CAD build for the part. Positions are in the model's coordinates, mm. Face numbers are marked on the shaded views. A direction names the side the tool comes from. Give positions to 0.01 mm unless a question says otherwise; leave off trailing zeros. Loops run counter-clockwise (first coordinate to the right, second up) from the corner with the lowest first, then second, coordinate; pieces in that order, holes last. Notation, with made-up numbers: (3, 20.5) - (22, 20.5) arc R19 cw to (22, 26.5) - close; hole circle Ø7 at (80, 20.25). An arc over 180 degrees is marked (long way). Return JSON: item names as keys, results as strings.
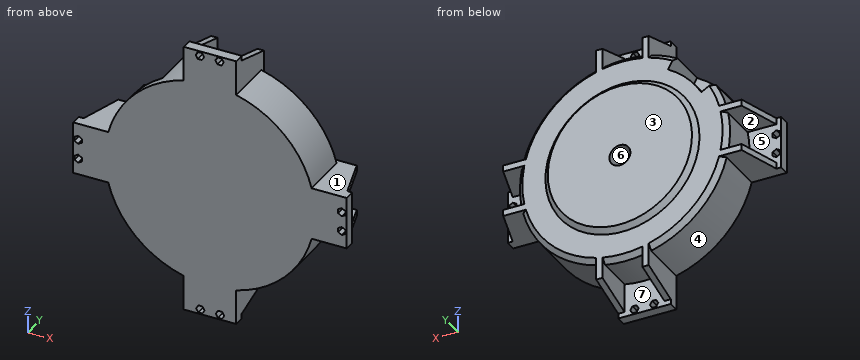
from build123d import *

# Parameters (mm, degrees)
BOSS_EXTRUDE1_DEPTH                      = 37.5
SKETCH4_W                                = 3.5
SKETCH4_H                                = 30
CUT_EXTRUDE1_DEPTH                       = 37.5
SKETCH7_W                                = 3.5
SKETCH7_H                                = 30
CUT_EXTRUDE3_DEPTH                       = 157.454118834
CUT_EXTRUDE4_START                       = -30
CUT_EXTRUDE4_DEPTH                       = 30
CHAMFER1_SIZE                            = 3.5
CUT_EXTRUDE5_DEPTH                       = 157.454118834
MIRROR4_AT_THE_SECOND_PLANE_COPY_1_DEPTH = 157.454118834
CUT_EXTRUDE6_DEPTH                       = 157.454118834
CUT_EXTRUDE7_DEPTH                       = 144.057956088
CUT_EXTRUDE7_DEPTH_BACK                  = 30
SKETCH14_R                               = 55
BOSS_EXTRUDE3_DEPTH                      = 3.5
CHAMFER2_SIZE                            = 3.5
SKETCH15_R                               = 7.5
CUT_EXTRUDE8_DEPTH                       = 25


with BuildPart() as part:
    # Sketch2 → Boss-Extrude1 (new body)
    with BuildSketch(Plane(origin=(0, 0, 0), x_dir=(1, 0, 0), z_dir=(0, 1, 0))):
        with BuildLine():
            Line((97.62, 0), (97.62, 18.75))
            Line((97.62, 18.75), (72.618437741, 18.75))
            ThreePointArc((72.618437741, 18.75), (53.033008589, 53.033008589), (18.75, 72.618437741))
            Line((18.75, 72.618437741), (18.75, 97.62))
            Line((18.75, 97.62), (0, 97.62))
            Line((0, 97.62), (-18.75, 97.62))
            Line((-18.75, 97.62), (-18.75, 72.618437741))
            ThreePointArc((-18.75, 72.618437741), (-53.033008589, 53.033008589), (-72.618437741, 18.75))
            Line((-72.618437741, 18.75), (-97.62, 18.75))
            Line((-97.62, 18.75), (-97.62, 0))
            Line((-97.62, 0), (-97.62, -18.75))
            Line((-97.62, -18.75), (-72.618437741, -18.75))
            ThreePointArc((-72.618437741, -18.75), (-53.033008589, -53.033008589), (-18.75, -72.618437741))
            Line((-18.75, -72.618437741), (-18.75, -97.62))
            Line((-18.75, -97.62), (0, -97.62))
            Line((0, -97.62), (18.75, -97.62))
            Line((18.75, -97.62), (18.75, -72.618437741))
            ThreePointArc((18.75, -72.618437741), (53.033008589, -53.033008589), (72.618437741, -18.75))
            Line((72.618437741, -18.75), (97.62, -18.75))
            Line((97.62, -18.75), (97.62, 0))
        make_face()
        Polygon((8.323894459, -96.71614814), (5.323896931, -96.72), (3.820562359, -94.12385186), (5.317225314, -91.52385186), (8.317222841, -91.52), (9.820557413, -94.11614814), align=None, mode=Mode.SUBTRACT)
        Polygon((-5.682777159, -96.72), (-4.179442587, -94.12385186), (-5.676105541, -91.52385186), (-8.676103069, -91.52), (-10.179437641, -94.11614814), (-8.682774686, -96.71614814), align=None, mode=Mode.SUBTRACT)
        Polygon((-96.71614814, -8.323894459), (-96.72, -5.323896931), (-94.12385186, -3.820562359), (-91.52385186, -5.317225314), (-91.52, -8.317222841), (-94.11614814, -9.820557413), align=None, mode=Mode.SUBTRACT)
        Polygon((96.72, -5.682777159), (94.12385186, -4.179442587), (91.52385186, -5.676105541), (91.52, -8.676103069), (94.11614814, -10.179437641), (96.71614814, -8.682774686), align=None, mode=Mode.SUBTRACT)
        Polygon((96.71614814, 8.323894459), (96.72, 5.323896931), (94.12385186, 3.820562359), (91.52385186, 5.317225314), (91.52, 8.317222841), (94.11614814, 9.820557413), align=None, mode=Mode.SUBTRACT)
        Polygon((-96.72, 5.682777159), (-94.12385186, 4.179442587), (-91.52385186, 5.676105541), (-91.52, 8.676103069), (-94.11614814, 10.179437641), (-96.71614814, 8.682774686), align=None, mode=Mode.SUBTRACT)
        Polygon((-8.323894459, 96.71614814), (-5.323896931, 96.72), (-3.820562359, 94.12385186), (-5.317225314, 91.52385186), (-8.317222841, 91.52), (-9.820557413, 94.11614814), align=None, mode=Mode.SUBTRACT)
        Polygon((5.682777159, 96.72), (4.179442587, 94.12385186), (5.676105541, 91.52385186), (8.676103069, 91.52), (10.179437641, 94.11614814), (8.682774686, 96.71614814), align=None, mode=Mode.SUBTRACT)
    extrude(amount=BOSS_EXTRUDE1_DEPTH)

    # Sketch4 → Cut-Extrude1 (cut)
    with BuildSketch(Plane.XY.offset(18.75)):
        with Locations((-95.87, 22.5)):
            Rectangle(SKETCH4_W, SKETCH4_H)
    cut_extrude1 = extrude(amount=-CUT_EXTRUDE1_DEPTH, mode=Mode.SUBTRACT)

    # Sketch7 → Cut-Extrude3 (cut, through all)
    with BuildSketch(Plane(origin=(18.75, 0, 0), x_dir=(0, 0, -1), z_dir=(1, 0, 0))):
        with Locations((-95.87, 22.5)):
            Rectangle(SKETCH7_W, SKETCH7_H)
    cut_extrude3 = extrude(amount=-CUT_EXTRUDE3_DEPTH, mode=Mode.SUBTRACT)

    # Mirror1: Cut-Extrude3 across plane
    add(cut_extrude3.mirror(Plane.XY), mode=Mode.SUBTRACT)

    # Mirror2: Cut-Extrude1 across plane
    add(cut_extrude1.mirror(Plane.ZY), mode=Mode.SUBTRACT)

    # Sketch8 → Cut-Extrude4 (cut)
    with BuildSketch(Plane(origin=(0, 37.5, 0), x_dir=(1, 0, 0), z_dir=(0, 1, 0)).offset(CUT_EXTRUDE4_START)):
        with BuildLine():
            Line((-14.25, 94.12), (-14.25, 73.633806774))
            ThreePointArc((-14.25, 73.633806774), (0, 75), (14.25, 73.633806774))
            Line((14.25, 73.633806774), (14.25, 94.12))
            Line((14.25, 94.12), (-14.25, 94.12))
        make_face()
        with BuildLine():
            Line((-94.12, 14.25), (-94.12, -14.25))
            Line((-94.12, -14.25), (-73.633806774, -14.25))
            ThreePointArc((-73.633806774, -14.25), (-75, 0), (-73.633806774, 14.25))
            Line((-73.633806774, 14.25), (-94.12, 14.25))
        make_face()
    cut_extrude4 = extrude(amount=CUT_EXTRUDE4_DEPTH, mode=Mode.SUBTRACT)

    # Mirror3: Cut-Extrude4 across plane
    add(cut_extrude4.mirror(Plane.ZY), mode=Mode.SUBTRACT)

    # Mirror3 at the second plane: Cut-Extrude4 across plane
    add(cut_extrude4.mirror(Plane.XY), mode=Mode.SUBTRACT)

    # Chamfer1
    chamfer1_edges = [part.edges().sort_by_distance(p)[0] for p in [
        (53.033008589, 37.5, -53.033008589),
        (0, 37.5, -75),
        (-75, 37.5, 0),
        (0, 37.5, 75),
        (-53.033008589, 37.5, -53.033008589),
        (75, 37.5, 0),
        (-53.033008589, 37.5, 53.033008589),
        (53.033008589, 37.5, 53.033008589),
    ]]
    chamfer(chamfer1_edges, length=CHAMFER1_SIZE)

    # Sketch9 → Cut-Extrude5 (cut, symmetric)
    with BuildSketch(Plane(origin=(18.75, 0, 0), x_dir=(0, 0, -1), z_dir=(1, 0, 0))):
        Polygon((-85.118437741, 37.5), (-94.12, 7.5), (-94.12, 37.5), align=None)
    cut_extrude5 = extrude(amount=CUT_EXTRUDE5_DEPTH, both=True, mode=Mode.SUBTRACT)

    # Mirror4: Cut-Extrude5 across plane
    add(cut_extrude5.mirror(Plane.ZY), mode=Mode.SUBTRACT)

    # Mirror4 at the second plane: Cut-Extrude5 across plane
    add(cut_extrude5.mirror(Plane.XY), mode=Mode.SUBTRACT)

    # Mirror4 at the second plane copy 1 sketc → Mirror4 at the second plane copy 1 (cut, symmetric)
    with BuildSketch(Plane.ZY.offset(18.75)):
        Polygon((-85.118437741, 37.5), (-94.12, 7.5), (-94.12, 37.5), align=None)
    extrude(amount=MIRROR4_AT_THE_SECOND_PLANE_COPY_1_DEPTH, both=True, mode=Mode.SUBTRACT)

    # Sketch10 → Cut-Extrude6 (cut, symmetric)
    with BuildSketch(Plane.XY.offset(18.75)):
        Polygon((-85.118437741, 37.5), (-94.12, 7.5), (-94.12, 37.5), align=None)
    cut_extrude6 = extrude(amount=CUT_EXTRUDE6_DEPTH, both=True, mode=Mode.SUBTRACT)

    # Mirror5: Cut-Extrude6 across plane
    add(cut_extrude6.mirror(Plane.ZY), mode=Mode.SUBTRACT)

    # Sketch11 → Cut-Extrude7 (cut, two sides: drawn at the far end of the back side and taken through both)
    with BuildSketch(Plane(origin=(0, 37.5, 0), x_dir=(1, 0, 0), z_dir=(0, 1, 0)).offset(-CUT_EXTRUDE7_DEPTH_BACK)):
        with BuildLine():
            Line((-56.291651246, -32.5), (-64.951905284, -37.5))
            ThreePointArc((-64.951905284, -37.5), (-53.033008589, -53.033008589), (-37.5, -64.951905284))
            Line((-37.5, -64.951905284), (-32.5, -56.291651246))
            ThreePointArc((-32.5, -56.291651246), (-45.961940777, -45.961940777), (-56.291651246, -32.5))
        make_face()
    extrude(amount=CUT_EXTRUDE7_DEPTH + CUT_EXTRUDE7_DEPTH_BACK, mode=Mode.SUBTRACT)

    # Sketch14 → Boss-Extrude3 (add)
    with BuildSketch(Plane(origin=(0, 37.5, 0), x_dir=(1, 0, 0), z_dir=(0, 1, 0))):
        with Locations(Location((0, 0, 0), (0, 0, 270))):
            Circle(SKETCH14_R)
    extrude(amount=BOSS_EXTRUDE3_DEPTH)

    # Chamfer2
    chamfer2_edges = [part.edges().sort_by_distance(p)[0] for p in [
        (0, 41, -55),
    ]]
    chamfer(chamfer2_edges, length=CHAMFER2_SIZE - 0.0001)  # a hair under: the kernel refuses the full size

    # Sketch15 → Cut-Extrude8 (cut)
    with BuildSketch(Plane(origin=(0, 41, 0), x_dir=(1, 0, 0), z_dir=(0, 1, 0))):
        with Locations(Location((0, 0, 0), (0, 0, 270))):
            Circle(SKETCH15_R)
    extrude(amount=-CUT_EXTRUDE8_DEPTH, mode=Mode.SUBTRACT)


solid = part.part
1. Drill centre lines: probe 1 along Z at (x, y) = (81, 19); probe 2 along X at (y, z) = (32.5, -0.5). Where is each one in solid material? Low to high.
Values follow:
{"probe 1": "z = -18.75 to -14.25, 14.25 to 18.75", "probe 2": "x = -75 to -7.48, 7.48 to 75"}
2. Which spindle directions (+Z, -Z, +X, -X, +Y, -Y) get a long thin tool onto all of the face, cutting with end or side? Do the marked faces 4, 5, 6 and 7. Say none if no direction does.
Values follow:
{"face 4": "-Z, -X, +Y, -Y", "face 5": "-X, +Y", "face 6": "+Y", "face 7": "-Z, +Y"}
3. Drop flat-ended pins along their axis: P1, Ø12, axis at x = -3.5, z = 85.5, coming from the +Y side; P2, Ø5, axis at x = 8, y = 33, coming from the -Z side; P3, Ø19, axis at x = -83.5, y = 15, coming from the -Z side; P4, Ø1.5, axis at x = 53.5, z = 18, coming from the -Y side. Give the stop position or say it passes through.
Values follow:
{"P1": "stops at y = 7.5", "P2": "stops at z = -74.8", "P3": "stops at z = -18.75", "P4": "stops at y = 0"}
4. Pull direction Z, two halves, no side cores. Call the marked faces 1, 2 and 3: +Z half, -Z half, draft (parallel to the pull), parting line (faces both ways), or undercut.
Values follow:
{"face 1": "+Z half", "face 2": "undercut", "face 3": "draft"}
5. Cut at D-D, the plane z = -79. Write the cut outline in (x, y).
Values follow:
{"outline": "(-18.75, 0) - (18.75, 0) - (18.75, 37.5) - (14.25, 37.5) - (14.25, 7.5) - (-14.25, 7.5) - (-14.25, 37.5) - (-18.75, 37.5) - close"}
6. Cut at C-C, the plane y = 5. Give the number of separate pieces and of enclosed holes in the cut face, plus the area to 3 significant figures.
Values follow:
{"separate pieces": "1", "enclosed holes": "8", "area": "21,000 mm²"}
